Design review of the part built by this model. Coordinates are the model's own, in mm. A direction names the side the tool comes from. Round coordinates to 2 decimals unless told otherwise and drop trailing zeros. Order: outer loops, then holes, each group sorted by start corner. A loop starts at its lowest first (then second) coordinate and runs counter-clockwise, first axis right, second up. Notation, with made-up numbers: M 21,2 L 50,2 A20 ccw 50,13 Z; hole C 79,88 d6. An arc over 180 degrees is marked long. Write each question's results on one line, items separated by ' | '. Start each with the question number.
Item 1: Take a section at B-B, the plane x = 144. Write out the cut boundary in (y, z).
Item 2: Machinability: for faces 1 (the flat face through (-11.019, -20.987, 1.972)), 2 (the cylindrical face through (123.18, 0.24, 1.97)), 3 (the flat face through (81, -20, 2)), which of the approach directions +Z, -Z, +X, -X, +Y, -Y give a long, thin tool a straight path to every point of the face, cutting with its end or side? Answer none if there is none.
Item 3: Wall thickness on line 1 (Y direction, x = -1, z = 1.9); line 2 (Y direction, x = 38.5, z = 1.6); line 3 (X direction, y = 6, z = 3.1) (3 decimals): over which ranges is each line inside the solid? List them lowest first. Write a range as [from, to].
Item 4: Take a section at A-A, the plane y = 0. Write out the cut boundary in (x, z).
Item 5: Take a section at C-C, the plane z = 2.7. Count the separate pieces of the cut face and the enclosed holes in it, plus the area to 3 significant figures.
Item 6: The part is to be moulded in two halves that separate along X. For faces 4 (the cylindrical face through (-1, -34, 2)), 5 (the cylindrical face through (3.054, 1.277, 1.972)), 6 (the flat face through (6.556, -24.93, 1.972)), 7 (the cylindrical face through (12.832, -0.241, 1.972)), say which applies: +X half, -X half, draft (parallel to the pull), parting line (faces both ways), or undercut.
Item 7: Take a section at D-D, the plane x = 118. Write out the cut boundary in (y, z).
Item 8: Clearance check with flat-ended pins moving along their axes: pin 1 (1.5 mm diameter, centred on x = -1, y = 17.12, fed in from +Z); pin 2 (2 mm diameter, centred on x = 76, z = 1, fed in from -Y); pin 3 (6.5 mm diameter, centred on x = 155.83, y = 11.72, fed in from +Z); pin 4 (1.5 mm diameter, centred on y = -12.5, z = 3.5, fed in from +X). State where each tip first meets the part, or that it passes through.
```python
from build123d import *

# Parameters (mm, degrees)
SKETCH_1_R      = 4.25
SKETCH_1_R_2    = 8.75
SKETCH_1_R_3    = 2
SKETCH_1_R_4    = 1.25
EXTRUDE_1_DEPTH = 4


with BuildPart() as part:
    # 草图1 → 凸台-拉伸1 (new body)
    with BuildSketch(Plane.XY):
        with BuildLine():
            Line((-5, -30), (-17.208156126, -11.717323713))
            ThreePointArc((-17.208156126, -11.717323713), (-18.809358134, 9.10092099), (-1, 20))
            Line((-1, 20), (149.064295006, 20))
            ThreePointArc((149.064295006, 20), (169.064295006, 0), (149.064295006, -20))
            Line((149.064295006, -20), (10.014533743, -20))
            Line((10.014533743, -20), (3, -30))
            ThreePointArc((3, -30), (-1, -34), (-5, -30))
        make_face()
        with Locations((-1, 0)):
            Circle(SKETCH_1_R, mode=Mode.SUBTRACT)
        with Locations((149.064295006, 0)):
            Circle(SKETCH_1_R_2, mode=Mode.SUBTRACT)
        with Locations((135.534295006, 0)):
            Circle(SKETCH_1_R_3, mode=Mode.SUBTRACT)
        with Locations((155.829295006, 11.717323713)):
            Circle(SKETCH_1_R_3, mode=Mode.SUBTRACT)
        with Locations((155.829295006, -11.717323713)):
            Circle(SKETCH_1_R_3, mode=Mode.SUBTRACT)
        with Locations((-1, -30)):
            Circle(SKETCH_1_R_3, mode=Mode.SUBTRACT)
        with Locations((-1, 17.12)):
            Circle(SKETCH_1_R_4, mode=Mode.SUBTRACT)
        with BuildLine():
            Line((23.78352134, 10.95385289), (112.230567298, 10.95385289))
            ThreePointArc((112.230567298, 10.95385289), (123.184420188, 0), (112.230567298, -10.95385289))
            Line((112.230567298, -10.95385289), (23.78352134, -10.95385289))
            ThreePointArc((23.78352134, -10.95385289), (12.829668451, 0), (23.78352134, 10.95385289))
        make_face(mode=Mode.SUBTRACT)
    extrude(amount=EXTRUDE_1_DEPTH)


solid = part.part
```
Results list:
1) outline: M -20,0 L -7.14,0 L -7.14,4 L -20,4 Z; M 7.14,0 L 20,0 L 20,4 L 7.14,4 Z
2) face 1: +Z, -Z, -X, -Y | face 2: +Z, -Z | face 3: +Z, -Z, +X, -Y
3) line 1: [-34, -32], [-28, -4.25], [4.25, 15.87], [18.37, 20] | line 2: [-20, -10.95], [10.95, 20] | line 3: [-20.079, 14.619], [121.395, 142.695], [155.433, 168.143]
4) outline: M -21,0 L -5.25,0 L -5.25,4 L -21,4 Z; M 3.25,0 L 12.83,0 L 12.83,4 L 3.25,4 Z; M 123.18,0 L 133.53,0 L 133.53,4 L 123.18,4 Z; M 137.53,0 L 140.31,0 L 140.31,4 L 137.53,4 Z; M 157.81,0 L 169.06,0 L 169.06,4 L 157.81,4 Z
5) separate pieces: 1 | enclosed holes: 8 | area: 4,780 mm²
6) face 4: parting line | face 5: undercut | face 6: +X half | face 7: undercut
7) outline: M -20,0 L -9.31,0 L -9.31,4 L -20,4 Z; M 9.31,0 L 20,0 L 20,4 L 9.31,4 Z
8) pin 1: through | pin 2: y = -20 | pin 3: z = 4 | pin 4: x = 165.25
